Source: CAD feature listing. Evaluate the final solid. Frame: model axes, mm. A direction names the side the tool comes from. Give positions to 0.01 mm unless a question says otherwise; leave off trailing zeros. Loops run counter-clockwise (first coordinate to the right, second up) from the corner with the lowest first, then second, coordinate; pieces in that order, holes last.
from build123d import *

# Parameters (mm, degrees)
BOSS_EXTRU_1_DEPTH      = 4.25
BOSS_EXTRU_2_DEPTH      = 4.25
ESQUISSE2_R             = 2
ENL_V_MAT_EXTRU_1_DEPTH = 8.5
ESQUISSE3_W             = 2.5
ESQUISSE3_H             = 3
ESQUISSE3_W_2           = 3
ESQUISSE3_H_2           = 2.5
BOSS_EXTRU_3_DEPTH      = 8
ESQUISSE4_W             = 14
ESQUISSE4_H             = 5
BOSS_EXTRU_4_DEPTH      = 45
ESQUISSE5_R             = 1.5
ESQUISSE5_R_2           = 5
ENL_V_MAT_EXTRU_2_DEPTH = 5
CONG_1_R                = 3
ESQUISSE6_W             = 2
ESQUISSE6_H             = 20
ENL_V_MAT_EXTRU_4_DEPTH = 14


with BuildPart() as part:
    # Esquisse1 → Boss.-Extru.1 (new body, symmetric)
    with BuildSketch(Plane(origin=(0, 0, 0), x_dir=(1, 0, 0), z_dir=(0, 1, 0))):
        with BuildLine():
            Line((7.778174593, -2.75), (-7.778174593, -2.75))
            ThreePointArc((-7.778174593, -2.75), (0, -8.25), (7.778174593, -2.75))
        make_face()
        with BuildLine():
            Line((7.778174593, 2.75), (-7.778174593, 2.75))
            ThreePointArc((-7.778174593, 2.75), (-8.25, 0), (-7.778174593, -2.75))
            Line((-7.778174593, -2.75), (7.778174593, -2.75))
            ThreePointArc((7.778174593, -2.75), (8.131188117, -1.395091324), (8.25, 0))
            ThreePointArc((8.25, 0), (8.131188117, 1.395091324), (7.778174593, 2.75))
        make_face()
        with BuildLine():
            ThreePointArc((7.778174593, 2.75), (0, 8.25), (-7.778174593, 2.75))
            Line((-7.778174593, 2.75), (7.778174593, 2.75))
        make_face()
    extrude(amount=BOSS_EXTRU_1_DEPTH, both=True)

    # Esquisse1<3> → Boss.-Extru.2 (add)
    with BuildSketch(Plane(origin=(0, 0, 0), x_dir=(1, 0, 0), z_dir=(0, 1, 0))):
        with BuildLine():
            Line((-7.778174593, 2.75), (-11, 2.75))
            Line((-11, 2.75), (-11, -2.75))
            Line((-11, -2.75), (-7.778174593, -2.75))
            ThreePointArc((-7.778174593, -2.75), (-8.25, 0), (-7.778174593, 2.75))
        make_face()
        with BuildLine():
            Line((11, 2.75), (7.778174593, 2.75))
            ThreePointArc((7.778174593, 2.75), (8.131188117, 1.395091324), (8.25, 0))
            ThreePointArc((8.25, 0), (8.131188117, -1.395091324), (7.778174593, -2.75))
            Line((7.778174593, -2.75), (11, -2.75))
            Line((11, -2.75), (11, 2.75))
        make_face()
    extrude(amount=BOSS_EXTRU_2_DEPTH)

    # Esquisse2 → Enlèv. mat.-Extru.1 (cut)
    with BuildSketch(Plane(origin=(0, 4.25, 0), x_dir=(1, 0, 0), z_dir=(0, 1, 0))):
        with Locations((0, -5)):
            Circle(ESQUISSE2_R)
    extrude(amount=-ENL_V_MAT_EXTRU_1_DEPTH, mode=Mode.SUBTRACT)

    # Esquisse3 → Boss.-Extru.3 (add)
    with BuildSketch(Plane.XZ.offset(4.25)):
        with Locations((-2.75, -2.924762745)):
            Rectangle(ESQUISSE3_W, ESQUISSE3_H)
        with Locations((0, -0.174762745)):
            Rectangle(ESQUISSE3_W_2, ESQUISSE3_H_2)
        with Locations((0, -2.924762745)):
            Rectangle(ESQUISSE3_W_2, ESQUISSE3_H)
        with Locations((0, -5.674762745)):
            Rectangle(ESQUISSE3_W_2, ESQUISSE3_H_2)
        with Locations((2.75, -2.924762745)):
            Rectangle(ESQUISSE3_W, ESQUISSE3_H)
    extrude(amount=BOSS_EXTRU_3_DEPTH)

    # Esquisse4 → Boss.-Extru.4 (add)
    with BuildSketch(Plane(origin=(0, 4.25, 0), x_dir=(1, 0, 0), z_dir=(0, 1, 0))):
        Rectangle(ESQUISSE4_W, ESQUISSE4_H)
    extrude(amount=BOSS_EXTRU_4_DEPTH)

    # Esquisse5 → Enlèv. mat.-Extru.2 (cut)
    with BuildSketch(Plane.XY.offset(2.5)):
        with Locations((-4, 46.25)):
            Circle(ESQUISSE5_R)
        with Locations((4, 46.25)):
            Circle(ESQUISSE5_R)
        with Locations((-4, 39.60357113)):
            Circle(ESQUISSE5_R)
        with Locations((4, 39.60357113)):
            Circle(ESQUISSE5_R)
        with Locations((0, 22.25)):
            Circle(ESQUISSE5_R_2)
        with Locations((-4, 12.278847644)):
            Circle(ESQUISSE5_R)
        with Locations((4, 12.278847644)):
            Circle(ESQUISSE5_R)
    extrude(amount=-ENL_V_MAT_EXTRU_2_DEPTH, mode=Mode.SUBTRACT)

    # Congé1
    cong_1_edges = [part.edges().sort_by_distance(p)[0] for p in [
        (-7, 49.25, 0),
        (7, 49.25, 0),
    ]]
    fillet(cong_1_edges, radius=CONG_1_R)

    # Esquisse6 → Enlèv. mat.-Extru.4 (cut)
    with BuildSketch(Plane(origin=(7, 0, 0), x_dir=(0, 0, -1), z_dir=(1, 0, 0))):
        with Locations((-1.5, 39.25)):
            Rectangle(ESQUISSE6_W, ESQUISSE6_H)
    extrude(amount=-ENL_V_MAT_EXTRU_4_DEPTH, mode=Mode.SUBTRACT)


solid = part.part
1) Cut plane B-B (y = 1.5). Return loops of the section in (x, z).
Checks:
outline: (-11, -2.75) - (-7.78, -2.75) arc R8.25 ccw to (7.78, -2.75) - (11, -2.75) - (11, 2.75) - (7.78, 2.75) arc R8.25 ccw to (-7.78, 2.75) - (-11, 2.75) - close; hole circle Ø4 at (0, 5)
2) Cut plane A-A (x = 0). Return loops of the section in (y, z).
Checks:
outline: (-12.25, -6.92) - (-4.25, -6.92) - (-4.25, -8.25) - (4.25, -8.25) - (4.25, -2.5) - (17.25, -2.5) - (17.25, 2.5) - (4.25, 2.5) - (4.25, 3) - (-4.25, 3) - (-4.25, 1.08) - (-12.25, 1.08) - close; (-4.25, 7) - (4.25, 7) - (4.25, 8.25) - (-4.25, 8.25) - close; (27.25, -2.5) - (49.25, -2.5) - (49.25, 0.5) - (29.25, 0.5) - (29.25, 2.5) - (27.25, 2.5) - close
3) Pull-direction query (Y, two-part tool) for faces 1 (the cylindrical face through (5.386, 39.029, -0.979)), 2 (the flat face through (-9, 2, 2.75)), 3 (the flat face through (0, -12.25, -3)), 4 (the cylindrical face through (5.386, 11.704, 0.035)); classes: released by +Y, released by -Y, zero draft, split by the parting line, or undercut.
Checks:
face 1: undercut
face 2: zero draft
face 3: released by -Y
face 4: undercut
4) Contact query for flat-ended pins moving along their axis: P1, Ø2, axis at y = 2.5, z = 5, coming from the -X side; P2, Ø3.5, axis at x = 0.5, y = -9.5, coming from the -Z side; P3, Ø2, axis at x = -1.5, z = -4.5, coming from the +Y side; P4, Ø8, axis at x = 1.5, y = 7, coming from the +Z side. Output: stop coordinate, or through.
Checks:
P1: stops at x = -7.22
P2: stops at z = -6.92
P3: stops at y = 4.25
P4: stops at z = 8.25
5) Cut plane D-D (z = 5). Return loops of the section in (x, y).
Checks:
outline: (-6.56, -4.25) - (-2, -4.25) - (-2, 4.25) - (-6.56, 4.25) - close; (2, -4.25) - (6.56, -4.25) - (6.56, 4.25) - (2, 4.25) - close
6) Reachability of faces 5 (the flat face through (-1.5, -8, -6)), 6 (the flat face through (0, 39, 0.5)), 7 (the flat face through (1.5, -8, -6)), 8 (the flat face through (3.01, 26.44, -2.5)), 9 (the flat face through (-3, -8, -1.425)) from +Z, -Z, +X, -X, +Y, -Y: full face, straight path, thin tool, end or side. Return the list, or none.
Checks:
face 5: -Z, -X, -Y
face 6: +Z, +X, -X, +Y
face 7: -Z, +X, -Y
face 8: -Z, +X, -X, +Y
face 9: +Z, -X, -Y
7) Ray query, probe 1 along Y at (x, z) = (4, -1.15); probe 2 along Y at (x, z) = (-3, 2.25); probe 3 along Z at (x, y) = (2.25, 41). Return the intervals inside material, ascending.
Checks:
probe 1: y = -4.25 to 10.78, 13.78 to 19.25, 25.25 to 38.1, 41.1 to 44.75, 47.75 to 49.25
probe 2: y = -4.25 to 11.16, 13.4 to 18.25, 26.25 to 29.25
probe 3: z = -2.5 to 0.5
8) Cut plane C-C (y = 22.25). Return loops of the section in (x, z).
Checks:
outline: (-7, -2.5) - (-5, -2.5) - (-5, 2.5) - (-7, 2.5) - close; (5, -2.5) - (7, -2.5) - (7, 2.5) - (5, 2.5) - close
